```python
from build123d import *

# Parameters (mm, degrees)
SKETCH1_W           = 48
SKETCH1_H           = 48
BOSS_EXTRUDE1_DEPTH = 72.5
SKETCH2_W           = 48
SKETCH2_H           = 48
BOSS_EXTRUDE2_DEPTH = 7.5
FILLET1_R           = 24
SKETCH3_R           = 5
CUT_EXTRUDE1_DEPTH  = 15
SKETCH4_R           = 5
BOSS_EXTRUDE3_DEPTH = 7.5


with BuildPart() as part:
    # Sketch1 → Boss-Extrude1 (new, symmetric)
    with BuildSketch(Plane(origin=(0, 0, 0), x_dir=(1, 0, 0), z_dir=(0, 1, 0))):
        with Locations((24, 24)):
            Rectangle(SKETCH1_W, SKETCH1_H)
    extrude(amount=BOSS_EXTRUDE1_DEPTH, both=True)

    # Sketch2 → Boss-Extrude2 (add, symmetric)
    with BuildSketch(Plane.ZY):
        with Locations((-24, 48.5)):
            Rectangle(SKETCH2_W, SKETCH2_H)
        with Locations((-24, -48.5)):
            Rectangle(SKETCH2_W, SKETCH2_H)
    extrude(amount=BOSS_EXTRUDE2_DEPTH, both=True)

    # Fillet1
    fillet1_edges = [part.edges().sort_by_distance(p)[0] for p in [
        (48, 72.5, -24),
        (0, 0, -48),
        (20.25, 72.5, -48),
        (0, 0, 0),
        (-3.75, 24.5, -48),
        (-3.75, 24.5, 0),
        (-3.75, -24.5, 0),
        (-3.75, -24.5, -48),
        (20.25, -72.5, -48),
        (48, -72.5, -24),
        (20.25, -72.5, 0),
        (48, 0, -48),
        (48, 0, 0),
        (20.25, 72.5, 0),
    ]]
    fillet(fillet1_edges, radius=FILLET1_R - 0.0001)  # a hair under: the kernel refuses the full size

    # Sketch3 → Cut-Extrude1 (cut)
    with BuildSketch(Plane.ZY.offset(7.5)):
        with Locations((-24, -48.5)):
            Circle(SKETCH3_R)
    extrude(amount=-CUT_EXTRUDE1_DEPTH, mode=Mode.SUBTRACT)

    # Sketch4 → Boss-Extrude3 (add, symmetric)
    with BuildSketch(Plane.ZY.offset(7.5)):
        with Locations((-24, 48.5)):
            Circle(SKETCH4_R)
    extrude(amount=BOSS_EXTRUDE3_DEPTH, both=True)


solid = part.part
```
Verification items for the finished model (mm, model axes). A direction names the side the tool comes from. Round coordinates to 2 decimals unless told otherwise and drop trailing zeros. Order: outer loops, then holes, each group sorted by start corner. A loop starts at its lowest first (then second) coordinate and runs counter-clockwise, first axis right, second up. Notation, with made-up numbers: (33, 75) - (92, 75) arc R9 ccw to (92, 91) - close; hole circle Ø6 at (35.5, 74.25). An arc over 180 degrees is marked (long way). Use CSV: the item, a comma, the result in double quotes. Start each with the question number.
1) Section check A-A, the plane x = -5. State how many separate pieces and enclosed holes the cut face has, plus the area to 3 significant figures.
2) Section check B-B, the plane z = -33. Record the cut outline in (x, y), plus the area to 3 significant figures.
3) Access from +Z, -Z, +X, -X, +Y, -Y to the whole of each face (thin tool, end or side, straight path). Record for faces 1 (the cylindrical face through (10.45, -0.68, -43.81)), 2 (the flat face through (-7.5, -48, -30)), 3 (the flat face through (7.5, -48, -24)), 4 (the cylindrical face through (1.03, 34.95, -4.19)).
4) Mould release check, pull along Y, two halves, no side actions. Record for faces 5 (the cylindrical face through (8.47, -65.66, -40.78)), 6 (the cylindrical face through (-0.105, -43.543, -24.651)), 7 (the cylindrical face through (40.78, -0.68, -41.16)): +Y half, -Y half, draft (parallel to the pull), parting line (faces both ways), or undercut.
5) Thickness scan on L1, parallel to Y at x = -2, z = -24; L2, parallel to Y at x = 3, z = -24; L3, parallel to Z at x = 2, y = -48. Record the ranges inside material, lowest first.
6) Go/stop test with flat-tipped pins: P1, Ø12, axis at x = -3, y = 50, coming from the +Z side; P2, Ø2, axis at x = 24.5, z = -28, coming from the -Y side; P3, Ø10, axis at y = -43, z = -12, coming from the -X side; P4, Ø1, axis at y = -56.5, z = -10, coming from the +X side. Record where each tip stops, or that it passes through.
Answers:
1,separate pieces,"2"
1,enclosed holes,"1"
1,area,"3,540 mm²"
2,outline,"(-7.5, -70.75) - (24, -70.75) arc R22.25 ccw to (46.25, -48.5) - (46.25, 48.5) arc R22.25 ccw to (24, 70.75) - (-7.5, 70.75) - (-7.5, 26.25) - (1.75, 26.25) - (1.75, -26.25) - (-7.5, -26.25) - close"
2,area,"6,910 mm²"
3,face 1,"-Z, -X"
3,face 2,"+Z, -Z, -X, -Y"
3,face 3,"-X"
3,face 4,"+Z, -X"
4,face 5,"-Y half"
4,face 6,"undercut"
4,face 7,"draft"
5,L1,"y = -72.5 to -53.5, -43.5 to -24.5, 24.5 to 72.5"
5,L2,"y = -72.5 to -53.5, -43.5 to 72.5"
5,L3,"z = -47.99 to -28.97, -19.03 to -0.01"
6,P1,"stops at z = 0"
6,P2,"stops at y = -72.31"
6,P3,"stops at x = -7.5"
6,P4,"stops at x = 42.22"
